Model file for the job. Use its own axes, mm. Round coordinates to 2 decimals unless told otherwise and drop trailing zeros. Loops run counter-clockwise (first coordinate to the right, second up) from the corner with the lowest first, then second, coordinate; pieces in that order, holes last. Notation, with made-up numbers: (31.25, 21) - (48.25, 21) arc R16 ccw to (48.25, 39) - close; hole circle Ø4 at (53, 18). An arc over 180 degrees is marked (long way). Answer as a JSON object with one key per item and string values.
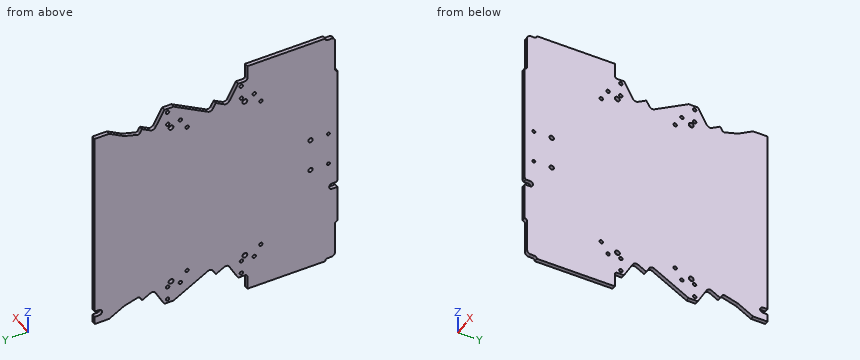
Autodesk Inventor part; units mm, degrees
ref_plane "LPmitBASE_XY" through (0, 0, 0) normal (1, 0, 0) x (0, 0, -1)
ref_plane "LPmitBASE_YZ" through (0, 0, 0) normal (0, 0, -1) x (0, 1, 0)
ref_plane "LPmitBASE_ZX" through (0, 0, 0) normal (0, 1, 0) x (1, 0, 0)
sketch "Sketch_2" plane through (0, 0, 0) normal (1, 0, 0) x (0, 1, 0)
  arc A0 (6, 49.5) -> (7, 50.5) centre (6, 50.5) ccw
  line L0 (6, 49.5) -> (4.5, 49.5)
  arc A1 (4.5, 49.5) -> (3, 48) centre (4.5, 48) ccw
  line L1 (3, 48) -> (3, 35)
  arc A2 (2, 34) -> (3, 35) centre (2, 35) ccw
  line L2 (2, 34) -> (2, -15.6072)
  line L3 (2, -15.6072) -> (2.4, -16.3)
  line L4 (2.4, -16.3) -> (4.2, -16.3)
  arc A3 (4.2, -18.7) -> (4.2, -16.3) centre (4.2, -17.5) ccw
  line L5 (4.2, -18.7) -> (2, -18.7)
  line L6 (2, -18.7) -> (2, -34)
  arc A4 (3, -35) -> (2, -34) centre (2, -35) ccw
  line L7 (3, -35) -> (3, -48)
  arc A5 (3, -48) -> (4.5, -49.5) centre (4.5, -48) ccw
  line L8 (4.5, -49.5) -> (6, -49.5)
  arc A6 (7, -50.5) -> (6, -49.5) centre (6, -50.5) ccw
  line L9 (7, -50.5) -> (38.7662, -50.5)
  line L10 (38.7662, -50.5) -> (38.7662, -45)
  arc A7 (39.7662, -44) -> (38.7662, -45) centre (39.7662, -45) ccw
  line L11 (39.7662, -44) -> (42.5044, -44)
  line L12 (42.5044, -44) -> (46.1424, -37.5038)
  arc A8 (48.1841, -36.928) -> (46.1424, -37.5038) centre (47.4512, -38.2367) ccw
  line L13 (48.1841, -36.928) -> (51.6116, -38.8475)
  line L14 (51.6116, -38.8475) -> (52.8016, -36.7226)
  arc A9 (54.8433, -36.1468) -> (52.8016, -36.7226) centre (54.1103, -37.4555) ccw
  line L15 (54.8433, -36.1468) -> (68.8661, -44)
  line L16 (68.8661, -44) -> (72.6044, -44)
  line L17 (72.6044, -44) -> (76.2424, -37.5038)
  arc A10 (78.2841, -36.928) -> (76.2424, -37.5038) centre (77.5512, -38.2367) ccw
  line L18 (78.2841, -36.928) -> (81.7116, -38.8475)
  line L19 (81.7116, -38.8475) -> (82.4858, -37.4651)
  arc A11 (82.7791, -37.1385) -> (82.4858, -37.4651) centre (83.3583, -37.9537) ccw
  arc A12 (83.6381, -36.9937) -> (82.7791, -37.1385) centre (83.3583, -37.9537) ccw
  line L20 (83.6381, -36.9937) -> (88.8034, -38.4993)
  arc A13 (89.1166, -38.6306) -> (88.8034, -38.4993) centre (88.3836, -39.9393) ccw
  line L21 (89.1166, -38.6306) -> (95.1331, -42)
  line L22 (95.1331, -42) -> (101, -42)
  line L23 (101, -42) -> (101, -38.75)
  line L24 (101, -38.75) -> (99.2, -38.75)
  arc A14 (98.4063, -38.45) -> (99.2, -38.75) centre (99.2, -37.55) ccw
  arc A15 (98.4063, -36.65) -> (98.4063, -38.45) centre (99.2, -37.55) ccw
  arc A16 (99.2, -36.35) -> (98.4063, -36.65) centre (99.2, -37.55) ccw
  line L25 (99.2, -36.35) -> (101, -36.35)
  line L26 (101, -36.35) -> (101, 42)
  line L27 (101, 42) -> (95.1331, 42)
  line L28 (95.1331, 42) -> (89.1166, 38.6306)
  arc A17 (88.8034, 38.4993) -> (89.1166, 38.6306) centre (88.3836, 39.9393) ccw
  line L29 (88.8034, 38.4993) -> (83.6381, 36.9937)
  arc A18 (82.7791, 37.1385) -> (83.6381, 36.9937) centre (83.3583, 37.9537) ccw
  arc A19 (82.4858, 37.4651) -> (82.7791, 37.1385) centre (83.3583, 37.9537) ccw
  line L30 (82.4858, 37.4651) -> (81.7116, 38.8475)
  line L31 (81.7116, 38.8475) -> (78.2841, 36.928)
  arc A20 (76.2424, 37.5038) -> (78.2841, 36.928) centre (77.5512, 38.2367) ccw
  line L32 (76.2424, 37.5038) -> (72.6044, 44)
  line L33 (72.6044, 44) -> (68.8661, 44)
  line L34 (68.8661, 44) -> (54.8433, 36.1468)
  arc A21 (52.8016, 36.7226) -> (54.8433, 36.1468) centre (54.1103, 37.4555) ccw
  line L35 (52.8016, 36.7226) -> (51.6116, 38.8475)
  line L36 (51.6116, 38.8475) -> (48.1841, 36.928)
  arc A22 (46.1424, 37.5038) -> (48.1841, 36.928) centre (47.4512, 38.2367) ccw
  line L37 (46.1424, 37.5038) -> (42.5044, 44)
  line L38 (42.5044, 44) -> (39.7662, 44)
  arc A23 (38.7662, 45) -> (39.7662, 44) centre (39.7662, 45) ccw
  line L39 (38.7662, 45) -> (38.7662, 50.5)
  line L40 (38.7662, 50.5) -> (7, 50.5)
  circle A24 centre (41.2057, -42.3862) radius 0.7
  circle A25 centre (71.3057, -42.3862) radius 0.7
  circle A26 centre (41.1709, -36.9226) radius 0.7
  circle A27 centre (71.2709, -36.9226) radius 0.7
  circle A28 centre (35.9795, -36.8806) radius 0.7
  circle A29 centre (66.0795, -36.8806) radius 0.7
  circle A30 centre (39.7889, -34.8879) radius 1
  circle A31 centre (69.8889, -34.8879) radius 1
  circle A32 centre (33.2312, -32.4762) radius 0.7
  circle A33 centre (63.3312, -32.4762) radius 0.7
  circle A34 centre (5.71, -6.75) radius 0.6
  circle A35 centre (13.01, -6.75) radius 0.9
  circle A36 centre (5.71, 6.75) radius 0.6
  circle A37 centre (13.01, 6.75) radius 0.9
  circle A38 centre (63.3312, 32.4762) radius 0.7
  circle A39 centre (33.2312, 32.4762) radius 0.7
  circle A40 centre (69.8889, 34.8879) radius 1
  circle A41 centre (39.7889, 34.8879) radius 1
  circle A42 centre (66.0795, 36.8806) radius 0.7
  circle A43 centre (35.9795, 36.8806) radius 0.7
  circle A44 centre (71.2709, 36.9226) radius 0.7
  circle A45 centre (41.1709, 36.9226) radius 0.7
  circle A46 centre (71.3057, 42.3862) radius 0.7
  circle A47 centre (41.2057, 42.3862) radius 0.7
extrude "Extrusion1" add sketch "Sketch_2" along normal blind 1.6
ref_plane "LPmitBASE_XY" through (0, 0, 0) normal (1, 0, 0) x (0, 0, -1)
ref_plane "LPmitBASE_YZ" through (0, 0, 0) normal (0, 0, -1) x (0, 1, 0)
ref_plane "LPmitBASE_ZX" through (0, 0, 0) normal (0, 1, 0) x (1, 0, 0)
ref_plane "mitSHL01_XY" through (0, 41.2057, -42.3862) normal (1, 0, 0) x (0, 0, -1)
ref_plane "mitSHL01_YZ" through (0, 41.2057, -42.3862) normal (0, 0, -1) x (0, 1, 0)
ref_plane "mitSHL01_ZX" through (0, 41.2057, -42.3862) normal (0, 1, 0) x (1, 0, 0)
ref_plane "mitSHL02_XY" through (0, 71.3057, -42.3862) normal (1, 0, 0) x (0, 0, -1)
ref_plane "mitSHL02_YZ" through (0, 71.3057, -42.3862) normal (0, 0, -1) x (0, 1, 0)
ref_plane "mitSHL02_ZX" through (0, 71.3057, -42.3862) normal (0, 1, 0) x (1, 0, 0)
ref_plane "mitSHL03_XY" through (0, 41.2057, 42.3862) normal (1, 0, 0) x (0, 0, -1)
ref_plane "mitSHL03_YZ" through (0, 41.2057, 42.3862) normal (0, 0, -1) x (0, 1, 0)
ref_plane "mitSHL03_ZX" through (0, 41.2057, 42.3862) normal (0, 1, 0) x (1, 0, 0)
ref_plane "mitSHL04_XY" through (0, 71.3057, 42.3862) normal (1, 0, 0) x (0, 0, -1)
ref_plane "mitSHL04_YZ" through (0, 71.3057, 42.3862) normal (0, 0, -1) x (0, 1, 0)
ref_plane "mitSHL04_ZX" through (0, 71.3057, 42.3862) normal (0, 1, 0) x (1, 0, 0)
properties part number "LP CH20M 5.0 2 PCB_5-2"
1) Slice it at A-A on z = -17.5. List the corners of the cut face in (x, y).
Values follow:
{"outline": "(0, 5.4) - (1.6, 5.4) - (1.6, 101) - (0, 101) - close"}
2) Drop flat-ended pins along their axis: P1, Ø0.8, axis at x = 1, y = 100, coming from the -Z side; P2, Ø0.8, axis at x = 1, z = 47.5, coming from the +Y side; P3, Ø0.5, axis at x = 1, y = 70, coming from the +Z side. Give the stop position or say it passes through.
Values follow:
{"P1": "z = -42", "P2": "y = 38.77", "P3": "z = 44"}
3) Probe probe 1 along Y at (x, z) = (0.8, -32.5); probe 2 along Z at (x, y) = (1.2, 70); probe 3 along Z at (x, y) = (0.5, 13.01). List the from-to ranges inside material, lowest first.
Values follow:
{"probe 1": "2 to 32.53, 33.93 to 62.63, 64.03 to 101", "probe 2": "-44 to -35.88, -33.89 to 33.89, 35.88 to 44", "probe 3": "-50.5 to -7.65, -5.85 to 5.85, 7.65 to 50.5"}
4) Slice it at B-B on x = 0.6. Count the separate pieces of the cut face and the enclosed holes in it, then the cut area to 3 significant figures.
Values follow:
{"separate pieces": "1", "enclosed holes": "24", "area": "8,580 mm²"}
